Model file for the job. Use its own axes, mm. A direction names the side the tool comes from. Round coordinates to 2 decimals unless told otherwise and drop trailing zeros. Order: outer loops, then holes, each group sorted by start corner. A loop starts at its lowest first (then second) coordinate and runs counter-clockwise, first axis right, second up. Notation, with made-up numbers: M 60,-29 L 111,-29 A18 cw 111,-12 Z; hole C 2.5,72 d2. An arc over 180 degrees is marked long. Return JSON: item names as keys, results as strings. Group by question number.
Item 1: Slice it at D-D on y = 0. Give the number of separate pieces and of enclosed holes in the cut face, then the cut area to 3 significant figures.
Item 2: Which spindle directions (+Z, -Z, +X, -X, +Y, -Y) get a long thin tool onto all of the face, cutting with end or side? Do faces 4 (the face through (18, -8, 493)), 5 (the face through (20, 9, 493)). Say none if no direction does.
Item 3: Pin check, flat tips, straight feed: pin 1 Ø12 at (x, y) = (11.5, -2.5) entering from +Z; pin 2 Ø12 at (y, z) = (-8, 307) entering from -X; pin 3 Ø1 at (x, y) = (-19, -2) entering from -Z. Stop position of each tip, or through.
Item 4: Slice it at A-A on x = 10.5. Write the cut outline in (y, z).
Item 5: Slice it at C-C on z = 353. Write the cut outline in (x, y), then the cut area to 3 significant figures.
Item 6: Pull direction Y, two halves, no side cores. Call faces 1 (the face through (19.01, 3, 890.46)), 2 (the face through (0, -20, 493)), 3 (the face through (-2, -19, 1000)): pulls with the +Y half, pulls with the -Y half, needs draft (parallel to the pull), parting line crosses it, or undercut.
Item 7: Probe line 1 along X through (y, z) = (-5.5, 378); line 2 along Y through (x, z) = (18.65, 500). List the from-to ranges inside material, lowest first.
Item 8: Slice it at B-B on z = 900. Write the cut outline in (x, y).
from build123d import *

# Parameters (mm, degrees)
CROQUIS1_W            = 40
CROQUIS1_H            = 40
CROQUIS1_W_2          = 36
CROQUIS1_H_2          = 36
EXTRUIR_L_MINA1_DEPTH = 1000
CROQUIS2_R            = 10
EXTRUIR1_DEPTH        = 10
CROQUIS3_W            = 60
CROQUIS3_H            = 30
EXTRUIR2_DEPTH        = 10


with BuildPart() as part:
    # Croquis1 → Extruir-Lámina1 (new body)
    with BuildSketch(Plane.XY):
        Rectangle(CROQUIS1_W, CROQUIS1_H)
        Rectangle(CROQUIS1_W_2, CROQUIS1_H_2, mode=Mode.SUBTRACT)
    extrude(amount=EXTRUIR_L_MINA1_DEPTH)

    # Croquis2 → Extruir1 (cut)
    with BuildSketch(Plane(origin=(20, 0, 0), x_dir=(0, 0, -1), z_dir=(1, 0, 0))):
        with Locations((-500, 0)):
            Circle(CROQUIS2_R)
        with Locations((-300, 0)):
            Circle(CROQUIS2_R)
        with Locations((-100, 0)):
            Circle(CROQUIS2_R)
        with Locations((-700, 0)):
            Circle(CROQUIS2_R)
        with Locations((-900, 0)):
            Circle(CROQUIS2_R)
    extrude(amount=-EXTRUIR1_DEPTH, mode=Mode.SUBTRACT)

    # Croquis3 → Extruir2 (cut)
    with BuildSketch(Plane.ZY.offset(20)):
        with Locations((100, 0)):
            Rectangle(CROQUIS3_W, CROQUIS3_H)
        with Locations((300, 0)):
            Rectangle(CROQUIS3_W, CROQUIS3_H)
        with Locations((500, 0)):
            Rectangle(CROQUIS3_W, CROQUIS3_H)
        with Locations((700, 0)):
            Rectangle(CROQUIS3_W, CROQUIS3_H)
        with Locations((900, 0)):
            Rectangle(CROQUIS3_W, CROQUIS3_H)
    extrude(amount=-EXTRUIR2_DEPTH, mode=Mode.SUBTRACT)


solid = part.part
Output values:
{
 "1": {"separate pieces": "12", "enclosed holes": "0", "area": "3,200 mm²"},
 "2": {"face 4": "+Z, -Z", "face 5": "+Z, -Z, +X, +Y, -Y"},
 "3": {"pin 1": "through", "pin 2": "x = 18", "pin 3": "z = 0"},
 "4": {"outline": "M -20,0 L -18,0 L -18,1000 L -20,1000 Z; M 18,0 L 20,0 L 20,1000 L 18,1000 Z"},
 "5": {"outline": "M -20,-20 L 20,-20 L 20,20 L -20,20 Z; hole M -18,-18 L 18,-18 L 18,18 L -18,18 Z", "area": "304 mm²"},
 "6": {"face 1": "undercut", "face 2": "pulls with the -Y half", "face 3": "needs draft"},
 "7": {"line 1": "-20 to -18, 18 to 20", "line 2": "-20 to -10, 10 to 20"},
 "8": {"outline": "M -20,-20 L 20,-20 L 20,-10 L 18,-10 L 18,-18 L -18,-18 L -18,-15 L -20,-15 Z; M -20,15 L -18,15 L -18,18 L 18,18 L 18,10 L 20,10 L 20,20 L -20,20 Z"}
}
